from build123d import *

# Parameters (mm, degrees)
F0_W     = 150
F0_H     = 100
F1_DEPTH = 50
F2_R     = 15.05
F2_R_2   = 15.5
F2_R_3   = 17.5
F3_DEPTH = 30


with BuildPart() as f1:
    # F0 (on Top) → F1 (new body)
    with BuildSketch(Plane.XY):
        Rectangle(F0_W, F0_H)
    extrude(amount=F1_DEPTH)

    # F2 (on face) → F3 (cut)
    with BuildSketch(Plane.XY.offset(50)):
        with Locations((-43.700065, 23.309725)):
            Circle(F2_R)
        with Locations((0, 23.955417)):
            Circle(F2_R_2)
        with Locations((43.468519, 23.309725)):
            Circle(F2_R_3)
        Polygon((-61.944879, -34.990932), (-31.845553, -35.192401), (-46.720739, -9.024886), align=None)
        Polygon((-15.296724, -37.1452), (15.702391, -36.910988), (0, -10.182073), align=None)
        Polygon((28.591996, -38.232997), (63.57602, -37.175601), (45.168276, -7.407246), align=None)
    extrude(amount=-F3_DEPTH, mode=Mode.SUBTRACT)


solid = f1.part
Design review of the part built by this model. Coordinates are the model's own, in mm. A direction names the side the tool comes from. Coordinates: 2 decimals unless noted, no trailing zeros. Loops run counter-clockwise (first coordinate to the right, second up) from the corner with the lowest first, then second, coordinate; pieces in that order, holes last. Notation, with made-up numbers: (39, 4) - (80, 4) arc R24 cw to (80, 29) - close; hole circle Ø8 at (25, 79.5). An arc over 180 degrees is marked (long way). Use CSV: the item, a comma, the result in double quotes. Start each with the question number.
1. Add section A-A on z = 24. Give the boundary of the cut face in (x, y), plus the area to 3 significant figures.
2. For faces 4 (the flat face through (-39.18, -22.29, 35.21)), 5 (the flat face through (-1, 1, 0)), list the 3-axis set-ups (+Z, -Z, +X, -X, +Y, -Y) from which the entire face can be reached by the end or side of a thin tool; tool diameter is ignored.
3. Clearance check with a flat-ended pin moving along its axis: pin 1 (9 mm diameter, centred on x = -45, y = 22.5, fed in from +Z). State where the tip first meets the part, or that it passes through.
4. Add section C-C on y = 34. Give the boundary of the cut face in (x, z), plus the area to 3 significant figures.
5. Mouldability with a two-part tool opening along Y and no side actions: class faces 1 (the flat face through (-47, -25, 20)), 2 (the flat face through (-1, -50, 25)), 3 (the flat face through (75, -1, 25)) as released by +Y, released by -Y, zero draft, split by the parting line, or undercut.
6. Add section B-B on y = -17. Give the boundary of the cut face in (x, z), plus the area to 3 significant figures.
7. To check wall thickness, follow probe 1 along X at (y, z) = (-28, 28.5); probe 2 along X at (y, z) = (-26, 47); probe 3 along Y at (x, z) = (49.5, 36). State the ranges of each line that lie inside material, in increasing order.
Resolved:
1,outline,"(-75, -50) - (75, -50) - (75, 50) - (-75, 50) - close; hole (-61.94, -34.99) - (-31.85, -35.19) - (-46.72, -9.02) - close; hole circle Ø30.1 at (-43.7, 23.31); hole circle Ø31 at (0, 23.96); hole (-15.3, -37.15) - (15.7, -36.91) - (0, -10.18) - close; hole circle Ø35 at (43.47, 23.31); hole (28.59, -38.23) - (63.58, -37.18) - (45.17, -7.41) - close"
1,area,"11,200 mm2"
2,face 4,"+Z"
2,face 5,"-Z, +X, -X, +Y, -Y"
3,pin 1,"z = 20"
4,outline,"(-75, 0) - (75, 0) - (75, 50) - (57.32, 50) - (57.32, 20) - (29.61, 20) - (29.61, 50) - (11.8, 50) - (11.8, 20) - (-11.8, 20) - (-11.8, 50) - (-33.11, 50) - (-33.11, 20) - (-54.29, 20) - (-54.29, 50) - (-75, 50) - close"
4,area,"5,320 mm2"
5,face 1,"undercut"
5,face 2,"released by -Y"
5,face 3,"zero draft"
6,outline,"(-75, 0) - (75, 0) - (75, 50) - (51.1, 50) - (51.1, 20) - (40.01, 20) - (40.01, 50) - (4.01, 50) - (4.01, 20) - (-3.87, 20) - (-3.87, 50) - (-42.19, 50) - (-42.19, 20) - (-51.4, 20) - (-51.4, 50) - (-75, 50) - close"
6,area,"6,650 mm2"
7,probe 1,"-75 to -57.85, -35.93 to -10.11, 10.47 to 34.09, 57.9 to 75"
7,probe 2,"-75 to -56.67, -37.07 to -8.97, 9.29 to 35.17, 56.67 to 75"
7,probe 3,"-50 to -37.6, -14.41 to 6.88, 39.74 to 50"
